from build123d import *

# Parameters (mm, degrees)
SKETCH1_R              = 15
BODY_DEPTH             = 5
SKETCH2_R              = 15
SKETCH2_R_2            = 10
SLEW_BEARING_LIP_DEPTH = 2.5
SKETCH3_R              = 2.5
CUT_EXTRUDE2_DEPTH     = 22.794494718
SKETCH4_R              = 1
CUT_EXTRUDE3_DEPTH     = 22.794494718


with BuildPart() as part:
    # Sketch1 → body (new body)
    with BuildSketch(Plane.XY):
        Circle(SKETCH1_R)
    extrude(amount=BODY_DEPTH)

    # Sketch2 → slew bearing lip (cut)
    with BuildSketch(Plane(origin=(0, 0, 0), x_dir=(-1, 0, 0), z_dir=(0, 0, -1))):
        Circle(SKETCH2_R)
        Circle(SKETCH2_R_2, mode=Mode.SUBTRACT)
    extrude(amount=-SLEW_BEARING_LIP_DEPTH, mode=Mode.SUBTRACT)

    # Sketch3 → Cut-Extrude2 (cut, through all)
    with BuildSketch(Plane.XY.offset(5)):
        with Locations((-5, 5)):
            Circle(SKETCH3_R)
        with Locations((5, 5)):
            Circle(SKETCH3_R)
        with Locations((5, -5)):
            Circle(SKETCH3_R)
        with Locations((-5, -5)):
            Circle(SKETCH3_R)
    extrude(amount=-CUT_EXTRUDE2_DEPTH, mode=Mode.SUBTRACT)

    # Sketch4 → Cut-Extrude3 (cut, through all)
    with BuildSketch(Plane.XY.offset(5)):
        with Locations((0, 5)):
            Circle(SKETCH4_R)
        with Locations((5, 0)):
            Circle(SKETCH4_R)
        with Locations((0, -5)):
            Circle(SKETCH4_R)
        with Locations((-5, 0)):
            Circle(SKETCH4_R)
    extrude(amount=-CUT_EXTRUDE3_DEPTH, mode=Mode.SUBTRACT)


solid = part.part
Input: part model. Units: mm. Frame: model coordinates. A direction names the side the tool comes from. Round coordinates to 2 decimals unless told otherwise and drop trailing zeros. Loops run counter-clockwise (first coordinate to the right, second up) from the corner with the lowest first, then second, coordinate; pieces in that order, holes last. Notation, with made-up numbers: M 56,5 L 79,5 A15 cw 79,32 Z; hole C 0.25,-9.75 d8. An arc over 180 degrees is marked long. Answer as CSV lines item,"result". Start each with the question number.
(1) Draft query along Y for faces 1 (the cylindrical face through (-2.615, 5.751, 2.535)), 2 (the flat face through (-10, -3, 2.5)), 3 (the cylindrical face through (-14.985, 0.66, 3.732)), 4 (the cylindrical face through (0, 6, 3)). Return one class per face: released by +Y, released by -Y, zero draft, split by the parting line, or undercut.
(2) Section B-B, the plane z = 3.25. State how many separate pieces and enclosed holes the cut face has, plus the area to 3 significant figures.
(3) First-contact query: pin 1 (1 mm diameter, centred on x = -7.5, z = 4, fed in from -Y); pin 2 (1.2 mm diameter, centred on x = -5, y = 0, fed in from +Z); pin 3 (1.5 mm diameter, centred on y = -6.5, z = 2.5, fed in from -X); pin 4 (3 mm diameter, centred on x = 0, y = -5, fed in from -Z). Flat tips, straight axial feed; report the tip coordinate or a pass-through.
(4) Section D-D, the plane x = -5. Output: boundary loops of the cut face in (y, z), plus the area to 3 significant figures.
(5) Reachability of faces 5 (the cylindrical face through (7.385, 5.751, 2.535)), 6 (the cylindrical face through (2.17, -9.76, 1.23)) from +Z, -Z, +X, -X, +Y, -Y: full face, straight path, thin tool, end or side. Return the list, or none.
(6) Section A-A, the plane x = 0. Output: boundary loops of the cut face in (y, z).
(7) Line query: line 1 (Y direction, x = 0, z = 3.6); line 2 (Y direction, x = -6.25, z = 2.75); line 3 (X direction, y = -4.25, z = 1.05). Output: solid intervals per line, ascending. Write a range as [from, to].
Values found:
1,face 1,"undercut"
1,face 2,"zero draft"
1,face 3,"split by the parting line"
1,face 4,"undercut"
2,separate pieces,"1"
2,enclosed holes,"8"
2,area,"616 mm²"
3,pin 1,"stops at y = -13.27"
3,pin 2,"passes through"
3,pin 3,"stops at x = -13.85"
3,pin 4,"stops at z = 0"
4,outline,"M -14.14,2.5 L -8.66,2.5 L -8.66,0 L -7.5,0 L -7.5,5 L -14.14,5 Z; M -2.5,0 L -1,0 L -1,5 L -2.5,5 Z; M 1,0 L 2.5,0 L 2.5,5 L 1,5 Z; M 7.5,0 L 8.66,0 L 8.66,2.5 L 14.14,2.5 L 14.14,5 L 7.5,5 Z"
4,area,"54.0 mm²"
5,face 5,"+Z, -Z"
5,face 6,"-Z"
6,outline,"M -15,2.5 L -10,2.5 L -10,0 L -6,0 L -6,5 L -15,5 Z; M -4,0 L 4,0 L 4,5 L -4,5 Z; M 6,0 L 10,0 L 10,2.5 L 15,2.5 L 15,5 L 6,5 Z"
7,line 1,"y = [-15, -6], [-4, 4], [6, 15]"
7,line 2,"y = [-13.64, -7.17], [-2.83, 2.83], [7.17, 13.64]"
7,line 3,"x = [-9.05, -7.38], [-2.62, -0.66], [0.66, 2.62], [7.38, 9.05]"
